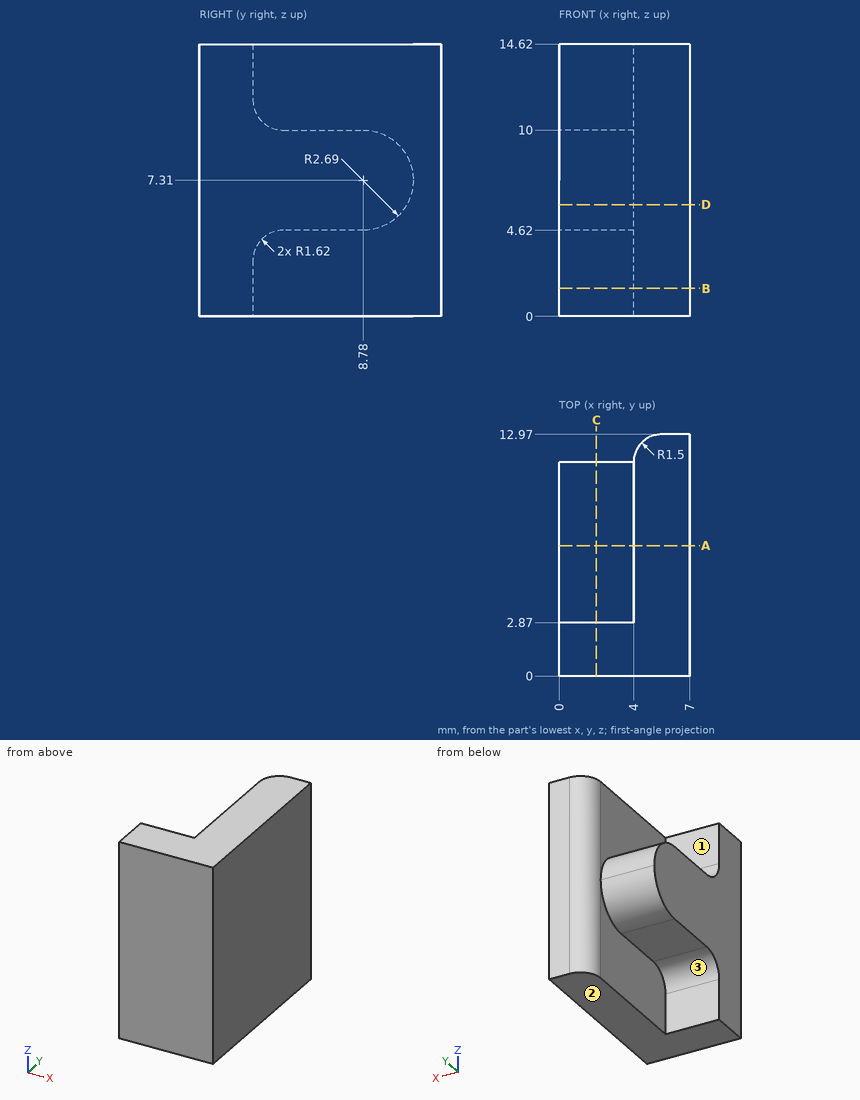
Check sheet for the drawn part. Datum: minimum x, y, z corner. Units: mm. A direction names the side the tool comes from. Coordinates: 2 decimals unless noted, no trailing zeros. Loops run counter-clockwise (first coordinate to the right, second up) from the corner with the lowest first, then second, coordinate; pieces in that order, holes last. Notation, with made-up numbers: (51, -11) -> (108, -11) arc R28 ccw to (108, 24) -> close; hole circle Ø11 at (83, -28). An arc over 180 degrees is marked (long way). Answer as a JSON object with one key per item and string values. Group by question number.
Item 1: Tool access check on the marked faces 1, 2 and 3. Record the directions out of +Z, -Z, +X, -X, +Y, -Y that give a thin tool (end or side, any length) a straight path to the whole face; none if there is none.
Item 2: Sectioned sample at D-D on z = 6. Record the boundary of the cut face in (x, y), plus the area to 3 significant figures.
Item 3: Sectioned sample at B-B on z = 1.5. Record the boundary of the cut face in (x, y), plus the area to 3 significant figures.
Item 4: Scan lines: probe 1 along X at (y, z) = (6, 12.5); probe 2 along Y at (x, z) = (1.25, 0.5); probe 3 along Z at (x, y) = (0.5, 6). Record each from-to range of solid material in increasing order.
Item 5: Depth check by flat-ended pin: pin 1 (3.5 mm diameter, centred on y = 8, z = 11.5, fed in from -X); pin 2 (3.5 mm diameter, centred on x = 3, z = 12.5, fed in from +Y); pin 3 (3.5 mm diameter, centred on x = 2, z = 2, fed in from +Y); pin 4 (1.2 mm diameter, centred on x = 2.5, y = 7, fed in from +Z). Enter the tip coordinate at first touch or a pass-through.
Item 6: Sectioned sample at C-C on x = 2. Record the boundary of the cut face in (y, z).
Item 7: Sectioned sample at A-A on y = 7. Record the boundary of the cut face in (x, z), plus the area to 3 significant figures.
Evaluation:
{
 "1": {"face 1": "+Z, -X, +Y", "face 2": "-Z, +X, -X, +Y, -Y", "face 3": "-Z, -X, +Y"},
 "2": {"outline": "(0, 0) -> (7, 0) -> (7, 12.97) -> (5.5, 12.97) arc R1.5 ccw to (4, 11.47) -> (4, 11.13) -> (0, 11.13) -> close", "area": "82.9 mm²"},
 "3": {"outline": "(0, 0) -> (7, 0) -> (7, 12.97) -> (5.5, 12.97) arc R1.5 ccw to (4, 11.47) -> (4, 2.87) -> (0, 2.87) -> close", "area": "49.9 mm²"},
 "4": {"probe 1": "x = 4 to 7", "probe 2": "y = 0 to 2.87", "probe 3": "z = 4.62 to 10"},
 "5": {"pin 1": "stops at x = 0", "pin 2": "stops at y = 12.77", "pin 3": "stops at y = 3.05", "pin 4": "stops at z = 10"},
 "6": {"outline": "(0, 0) -> (2.87, 0) -> (2.87, 3) arc R1.62 cw to (4.49, 4.62) -> (8.78, 4.62) arc R2.69 ccw to (8.78, 10) -> (4.49, 10) arc R1.62 cw to (2.87, 11.62) -> (2.87, 14.62) -> (0, 14.62) -> close"},
 "7": {"outline": "(0, 4.62) -> (4, 4.62) -> (4, 0) -> (7, 0) -> (7, 14.62) -> (4, 14.62) -> (4, 10) -> (0, 10) -> close", "area": "65.4 mm²"}
}
